Autodesk Inventor part; units mm, degrees
ref_plane "YZ Plane" through (0, 0, 0) normal (1, 0, 0) x (0, 1, 0)
ref_plane "XZ Plane" through (0, 0, 0) normal (0, 1, 0) x (-1, 0, 0)
ref_plane "XY Plane" through (0, 0, 0) normal (0, 0, 1) x (1, 0, 0)
sketch "Sketch1" plane through (0, 0, 0) normal (0, 0, 1) x (1, 0, 0)
  line L0 (0, 0) -> (0, 31.75)
  line L1 (0, 31.75) -> (57.15, 31.75)
  line L2 (57.15, 31.75) -> (57.15, 0)
  line L3 (53.975, 0) -> (53.975, 28.575)
  line L4 (53.975, 28.575) -> (3.175, 28.575)
  line L5 (3.175, 28.575) -> (3.175, 0)
  line L6 (0, 0) -> (3.175, 0)
  line L7 (53.975, 0) -> (57.15, 0)
  dimension "d0" = 31.75
  dimension "d1" = 31.75
  dimension "d2" = 57.15
  dimension "d3" = 3.175
extrude "Extrusion1" add sketch "Sketch1" along normal blind 38.1
sketch "Sketch2" plane through (57.15, 0, 0) normal (1, 0, 0) x (0, 0, -1)
  circle A0 centre (-19.05, 15.875) radius 9.525
  dimension "d6" = 19.05
extrude "Extrusion2" cut sketch "Sketch2" against normal blind 38.1
sketch "Sketch3" plane through (0, 0, 0) normal (-1, 0, 0) x (0, 0, 1)
  circle A0 centre (19.05, 15.875) radius 1.5875
  dimension "d10" = 3.175
extrude "Extrusion3" cut sketch "Sketch3" against normal blind 38.1
sketch "Sketch4" plane through (0, 31.75, 0) normal (0, 1, 0) x (1, 0, 0)
  line L0 (0, 0) -> (57.15, 0)
  line L1 (0, 0) -> (0, -38.1)
  line L2 (57.15, -38.1) -> (0, -38.1)
  line L3 (57.15, 0) -> (57.15, -38.1)
  circle A0 centre (10.16, -19.05) radius 1.5926
  circle A1 centre (46.99, -19.05) radius 1.5875
  circle A2 centre (28.575, -31.75) radius 1.5875
  circle A3 centre (28.575, -6.35) radius 1.5875
  dimension "d14" = 10.16
  dimension "d15" = 10.16
  dimension "d16" = 19.05
  dimension "d17" = 19.05
  dimension "d18" = 3.1852
  dimension "d19" = 3.175
  dimension "d20" = 3.175
  dimension "d21" = 6.35
  dimension "d22" = 6.35
  dimension "d23" = 3.175
extrude "Extrusion4" cut sketch "Sketch4" against normal blind 38.1 contours A0 | A1 | A2 | A3
sketch "Sketch5" plane through (57.15, 0, 0) normal (1, 0, 0) x (0, 0, -1)
  circle A0 centre (-19.05, 15.875) radius 9.525
extrude "Extrusion5" cut sketch "Sketch5" against normal blind 127
properties part number "Mount" material "Aluminum 6061"
Verification items for the finished model (mm, model axes). A direction names the side the tool comes from. Give positions to 0.01 mm unless a question says otherwise; leave off trailing zeros. Loops run counter-clockwise (first coordinate to the right, second up) from the corner with the lowest first, then second, coordinate; pieces in that order, holes last.
1. Set-up check for faces 4 (the flat face through (3.175, 11, 10)), 5 (the cylindrical face through (45.404, 30.185, 18.98)): record each of +Z, -Z, +X, -X, +Y, -Y from which the full face is reachable in a straight line by a thin tool's end or side.
2. Mould release check, pull along Z, two halves, no side actions. Record for faces 1 (the cylindrical face through (55.585, 18.736, 9.965)), 2 (the flat face through (53.975, 11, 10)), 3 (the flat face through (24, 29, 38.1)): released by +Z, released by -Z, zero draft, split by the parting line, or undercut.
3. Section check C-C, the plane z = 19.05. Count the separate pieces of the cut face and the enclosed holes in it, then the cut area to 3 significant figures.
4. Go/stop test with flat-tipped pins: pin 1 Ø15 at (y, z) = (15.875, 19.05) entering from +X; pin 2 Ø4 at (x, z) = (28.575, 31.75) entering from -Y (3 decimals). Record where each tip stops, or that it passes through.
5. Section check B-B, the plane x = 10.16. Enter the section's corners in (y, z) (3 decimals).
6. Thickness scan on line 1 (X direction, y = 29.7, z = 19.05); line 2 (X direction, y = 10, z = 33.5) (3 decimals); line 3 (Z direction, x = 28, y = 29). Record the ranges inside material, lowest first.
7. Section check D-D, the plane y = 14.5. Enter the section's corners in (x, z) (3 decimals), then the cut area to 3 significant figures.
Geometry says:
1. face 4: +Z, -Z, -Y
1. face 5: +Y, -Y
2. face 1: undercut
2. face 2: zero draft
2. face 3: released by +Z
3. separate pieces: 5
3. enclosed holes: 0
3. area: 222 mm2
4. pin 1: passes through
4. pin 2: stops at y = 28.575
5. outline: (28.575, 0) - (31.75, 0) - (31.75, 17.457) - (28.575, 17.457) - close; (28.575, 20.643) - (31.75, 20.643) - (31.75, 38.1) - (28.575, 38.1) - close
6. line 1: x = 0 to 8.57, 11.75 to 45.4, 48.58 to 57.15
6. line 2: x = 0 to 3.175, 53.975 to 57.15
6. line 3: z = 0 to 4.87, 7.83 to 30.27, 33.23 to 38.1
7. outline: (0, 0) - (3.175, 0) - (3.175, 9.625) - (0, 9.625) - close; (0, 28.475) - (3.175, 28.475) - (3.175, 38.1) - (0, 38.1) - close; (53.975, 0) - (57.15, 0) - (57.15, 9.625) - (53.975, 9.625) - close; (53.975, 28.475) - (57.15, 28.475) - (57.15, 38.1) - (53.975, 38.1) - close
7. area: 122 mm2
